```python
from build123d import *

# Parameters (mm, degrees)
SKETCH3_R                                         = 66.5
BOSS_EXTRUDE1_DEPTH                               = 2
CSK_FOR_M2_5_FLAT_HEAD_MACHINE_SCREW2_D           = 2.9
CSK_FOR_M2_5_FLAT_HEAD_MACHINE_SCREW2_DEPTH       = 2
CSK_FOR_M2_5_FLAT_HEAD_MACHINE_SCREW2_CSINK_D     = 5.5
CSK_FOR_M2_5_FLAT_HEAD_MACHINE_SCREW2_CSINK_ANGLE = 90
CSK_FOR_M2_5_FLAT_HEAD_MACHINE_SCREW2_TIP         = 0.871247898
SKETCH4_R                                         = 2.5
CUT_EXTRUDE1_DEPTH                                = 1
CIRPATTERN1_COUNT                                 = 4
SKETCH9_R                                         = 0.5
CUT_EXTRUDE2_DEPTH                                = 95.066465863
CIRPATTERN2_COUNT                                 = 9


with BuildPart() as part:
    # Sketch3 → Boss-Extrude1 (new body)
    with BuildSketch(Plane(origin=(0, 0, 0), x_dir=(1, 0, 0), z_dir=(0, 1, 0))):
        with Locations(Location((0, 0, 0), (0, 0, 270))):
            Circle(SKETCH3_R)
    extrude(amount=BOSS_EXTRUDE1_DEPTH)

    # CSK for M2.5 Flat Head Machine Screw2
    with Locations(Plane(origin=(0, 0, 0), x_dir=(-1, 0, 0), z_dir=(0, -1, 0))):
        with Locations((-60, 0), (0, 60), (60, 0), (0, -60)):
            CounterSinkHole(CSK_FOR_M2_5_FLAT_HEAD_MACHINE_SCREW2_D / 2, CSK_FOR_M2_5_FLAT_HEAD_MACHINE_SCREW2_CSINK_D / 2, depth=CSK_FOR_M2_5_FLAT_HEAD_MACHINE_SCREW2_DEPTH, counter_sink_angle=CSK_FOR_M2_5_FLAT_HEAD_MACHINE_SCREW2_CSINK_ANGLE)
            with Locations((0, 0, -(CSK_FOR_M2_5_FLAT_HEAD_MACHINE_SCREW2_DEPTH + CSK_FOR_M2_5_FLAT_HEAD_MACHINE_SCREW2_TIP / 2))):  # 118° drill point
                Cone(0, CSK_FOR_M2_5_FLAT_HEAD_MACHINE_SCREW2_D / 2, CSK_FOR_M2_5_FLAT_HEAD_MACHINE_SCREW2_TIP, mode=Mode.SUBTRACT)

    # Sketch4 → Cut-Extrude1 (cut)
    with BuildSketch(Plane(origin=(0, 0, 0), x_dir=(-1, 0, 0), z_dir=(0, -1, 0))):
        with Locations(Location((-38.890872965, 38.890872965, 0), (0, 0, 90))):
            Circle(SKETCH4_R)
    cut_extrude1 = extrude(amount=-CUT_EXTRUDE1_DEPTH, mode=Mode.SUBTRACT)

    # CirPattern1: Cut-Extrude1 ×4 about axis
    cirpattern1_axis = Axis((-0.05542221, 0, 0.05542221), (0, 1, 0))
    for i in range(1, CIRPATTERN1_COUNT):
        add(cut_extrude1.rotate(cirpattern1_axis, i * 360 / CIRPATTERN1_COUNT), mode=Mode.SUBTRACT)

    # Sketch9 → Cut-Extrude2 (cut, through all)
    with BuildSketch(Plane.XZ):
        with Locations(Location((0, 0, 0), (0, 0, 270))):
            Circle(SKETCH9_R)
        with Locations(Location((0, 3, 0), (0, 0, 270))):
            Circle(SKETCH9_R)
        with Locations(Location((0, 6, 0), (0, 0, 270))):
            Circle(SKETCH9_R)
    cut_extrude2 = extrude(amount=-CUT_EXTRUDE2_DEPTH, mode=Mode.SUBTRACT)

    # CirPattern2: Cut-Extrude2 ×9 about axis
    cirpattern2_axis = Axis((0, 0, 0), (0, 1, 0))
    for i in range(1, CIRPATTERN2_COUNT):
        add(cut_extrude2.rotate(cirpattern2_axis, i * 360 / CIRPATTERN2_COUNT), mode=Mode.SUBTRACT)


solid = part.part
```
Check sheet for the modelled part. Datum: model origin and axes. Units: mm. A direction names the side the tool comes from. Round coordinates to 2 decimals unless told otherwise and drop trailing zeros. Loops run counter-clockwise (first coordinate to the right, second up) from the corner with the lowest first, then second, coordinate; pieces in that order, holes last. Notation, with made-up numbers: (-2.75, 30.25) -> (4.25, 30.25) arc R25 ccw to (4.25, 54.25) -> close; hole circle Ø1 at (-2.5, 36). An arc over 180 degrees is marked (long way). Write item = value, one per line. Start each with the question number.
1) Sectioned sample at B-B, the plane x = -16.5. Record the cut outline in (y, z), plus the area to 3 significant figures.
2) Sectioned sample at C-C, the plane z = 28. Record the cut outline in (x, y), plus the area to 3 significant figures.
3) Gauge pin test, flat ends, axial feed: pin 1 Ø5.5 at (x, z) = (-39, -38) entering from -Y; pin 2 Ø4.5 at (x, z) = (-39, 39) entering from -Y; pin 3 Ø1 at (y, z) = (1, 17.5) entering from +X; pin 4 Ø4.5 at (x, z) = (60, 0) entering from -Y. Record the tip position at first contact, or that the pin passes through.
4) Sectioned sample at A-A, the plane y = 0.6. State how many separate pieces and enclosed holes the cut face has, plus the area to 3 significant figures.
5) Thickness scan on probe 1 along Z at (x, y) = (-40.5, 0.8); probe 2 along Z at (x, y) = (-59.5, 0.7); probe 3 along X at (y, z) = (1.5, -31.5). Record the ranges inside material, lowest first.
6) Set-up check for faces 1 (the flat face through (39, 1, -39)), 2 (the cylindrical face through (58.55, 1.65, -0.06)): record each of +Z, -Z, +X, -X, +Y, -Y from which the full face is reachable in a straight line by a thin tool's end or side.
7) Release check for a two-part mould opening along Z. For faces 3 (the cylindrical face through (65.934, 0.986, -8.657)), 4 (the flat face through (39, 1, 39)), 5 (the flat face through (1, 2, -1)) record: released by +Z, released by -Z, zero draft, split by the parting line, or undercut.
Results are:
q1.outline = (0, -64.42) -> (2, -64.42) -> (2, 64.42) -> (0, 64.42) -> close
q1.area = 258 mm^2
q2.outline = (-60.32, 0) -> (60.32, 0) -> (60.32, 2) -> (-60.32, 2) -> close
q2.area = 241 mm^2
q3.pin_1 = 0
q3.pin_2 = 1
q3.pin_3 = 64.29
q3.pin_4 = 0.5
q4.separate_pieces = 1
q4.enclosed_holes = 27
q4.area = 13,700 mm^2
q5.probe_1 = -52.74 to -40.89, -36.89 to 37, 41 to 52.74
q5.probe_2 = -29.7 to -1.99, 1.99 to 29.7
q5.probe_3 = -58.57 to 58.57
q6.face_1 = -Y
q6.face_2 = +Y, -Y
q7.face_3 = split by the parting line
q7.face_4 = undercut
q7.face_5 = zero draft
